```python
from build123d import *

# Parameters (mm, degrees)
BOSS_EXTRUDE1_DEPTH = 25.8


with BuildPart() as part:
    # Sketch1 → Boss-Extrude1 (new body)
    with BuildSketch(Plane.XZ.offset(25.8)):
        with BuildLine():
            Line((-0.494571956, -23.689779316), (-0.494571956, -23.589779316))
            Line((-0.494571956, -23.589779316), (-0.394571956, -23.589779316))
            Line((-0.394571956, -23.589779316), (33.993371563, -23.589779316))
            Line((33.993371563, -23.589779316), (38.063220374, -23.589779316))
            Line((38.063220374, -23.589779316), (37.29331502, -27.450677709))
            add(Edge.make_bspline(
                [(33.373472705, -47.107785962), (35.333393862, -37.279231836), (37.29331502, -27.450677709)],
                knots=[0, 0, 0, 1, 1, 1], degree=2))
            ThreePointArc((33.373472705, -47.107785962), (20.478962104, -86.002469597), (1.348099623, -122.238845235))
            Line((1.348099623, -122.238845235), (-0.494571956, -125.122735442))
            Line((-0.494571956, -125.122735442), (-0.494571956, -121.700417329))
            Line((-0.494571956, -121.700417329), (-0.494571956, -23.689779316))
        make_face()
        Polygon((1.636693568, -33.589779316), (31.180296724, -33.589779316), (28.552125449, -44.152877649), align=None, mode=Mode.SUBTRACT)
        with BuildLine():
            Line((1.8, -35.835600274), (27.903926427, -46.080219159))
            ThreePointArc((27.903926427, -46.080219159), (27.424243887, -48.283989571), (26.927669734, -50.484015362))
            Line((26.927669734, -50.484015362), (1.8, -38.383681926))
            Line((1.8, -38.383681926), (1.8, -35.835600274))
        make_face(mode=Mode.SUBTRACT)
        with BuildLine():
            Line((1.8, -40.603496686), (26.461878816, -52.479526576))
            ThreePointArc((26.461878816, -52.479526576), (25.912863392, -54.754715884), (25.345753049, -57.025462497))
            Line((25.345753049, -57.025462497), (1.8, -43.431924445))
            Line((1.8, -43.431924445), (1.8, -40.603496686))
        make_face(mode=Mode.SUBTRACT)
        with BuildLine():
            Line((1.8, -45.741299666), (24.827629624, -59.035712415))
            ThreePointArc((24.827629624, -59.035712415), (24.198120154, -61.402606851), (23.548915198, -63.764175052))
            Line((23.548915198, -63.764175052), (1.8, -48.936721812))
            Line((1.8, -48.936721812), (1.8, -45.741299666))
        make_face(mode=Mode.SUBTRACT)
        with BuildLine():
            Line((1.8, -51.35729301), (22.974243013, -65.792960045))
            ThreePointArc((22.974243013, -65.792960045), (22.250225593, -68.273323364), (21.504437212, -70.747227791))
            Line((21.504437212, -70.747227791), (1.8, -55.034267198))
            Line((1.8, -55.034267198), (1.8, -51.35729301))
        make_face(mode=Mode.SUBTRACT)
        with BuildLine():
            Line((1.8, -57.592312351), (20.868191148, -72.797909591))
            ThreePointArc((20.868191148, -72.797909591), (20.032066674, -75.415616602), (19.171511459, -78.02539415))
            Line((19.171511459, -78.02539415), (1.8, -61.907631839))
            Line((1.8, -61.907631839), (1.8, -57.592312351))
        make_face(mode=Mode.SUBTRACT)
        with BuildLine():
            Line((1.8, -63.544593475), (18.75085734, -79.272061417))
            ThreePointArc((18.75085734, -79.272061417), (17.733603559, -82.213523384), (16.685267787, -85.144051641))
            Line((16.685267787, -85.144051641), (1.8, -69.379364433))
            Line((1.8, -69.379364433), (1.8, -63.544593475))
        make_face(mode=Mode.SUBTRACT)
        with BuildLine():
            Line((1.8, -71.127270664), (16.223970717, -86.40340744))
            ThreePointArc((16.223970717, -86.40340744), (15.062552919, -89.498168213), (13.866413905, -92.579675475))
            Line((13.866413905, -92.579675475), (1.8, -77.977808183))
            Line((1.8, -77.977808183), (1.8, -71.127270664))
        make_face(mode=Mode.SUBTRACT)
        with BuildLine():
            Line((1.8, -79.861617911), (13.360943276, -93.851802636))
            ThreePointArc((13.360943276, -93.851802636), (12.031133738, -97.119012014), (10.66221999, -100.37003119))
            Line((10.66221999, -100.37003119), (1.8, -88.073893757))
            Line((1.8, -88.073893757), (1.8, -79.861617911))
        make_face(mode=Mode.SUBTRACT)
        with BuildLine():
            Line((1.8, -90.126243158), (10.108701369, -101.654385546))
            ThreePointArc((10.108701369, -101.654385546), (8.581699979, -105.113401186), (7.010340095, -108.552492716))
            Line((7.010340095, -108.552492716), (1.8, -100.212262217))
            Line((1.8, -100.212262217), (1.8, -90.126243158))
        make_face(mode=Mode.SUBTRACT)
        with BuildLine():
            Line((1.8, -102.47713769), (6.404592978, -109.847744231))
            ThreePointArc((6.404592978, -109.847744231), (4.143731804, -114.543136732), (1.8, -119.197717832))
            Line((1.8, -119.197717832), (1.8, -102.47713769))
        make_face(mode=Mode.SUBTRACT)
    extrude(amount=-BOSS_EXTRUDE1_DEPTH)


solid = part.part
```
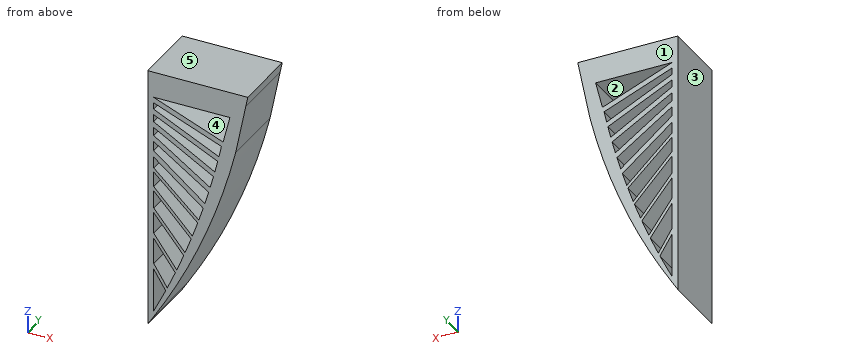
Geometry: final body of the model. Coordinates: model frame, mm. Face numbers are marked on the shaded views. A direction names the side the tool comes from. Round coordinates to 2 decimals unless told otherwise and drop trailing zeros. Order: outer loops, then holes, each group sorted by start corner. A loop starts at its lowest first (then second) coordinate and runs counter-clockwise, first axis right, second up. Notation, with made-up numbers: (70, 7.5) - (126, 7.5) arc R21 ccw to (126, 33.5) - close; hole circle Ø11 at (26.5, 89). An arc over 180 degrees is marked (long way). Use CSV: the item, a comma, the result in double quotes. Start each with the question number.
Q1. First-contact query: pin 1 (1.4 mm diameter, centred on y = -7.5, z = -42, fed in from +X); pin 2 (2 mm diameter, centred on y = -18.5, z = -37.5, fed in from +X); pin 3 (5.5 mm diameter, centred on y = -19.5, z = -76, fed in from +X); pin 4 (8 mm diameter, centred on x = 6, z = -50.5, fed in from +Y). Flat tips, straight axial feed; report the tip coordinate or a pass-through.
Q2. Section query A-A (x = 29.5). Return loops of the section in (y, z), and give its area (3 significant figures).
Q3. Mould query, pull axis X, two halves, no side actions, for the marked faces 3, 4 and 5. Classes: +X half, -X half, draft (parallel to the pull), parting line (faces both ways), or undercut.
Q4. Material intervals for line 1 along X through (y, z) = (-16.75, -97); line 2 along X through (y, z) = (-15.75, -66.5); line 3 along X through (y, z) = (-18, -94), sorted ascending. Write a range as from..to.
Q5. Section query B-B (z = -112.5). Return loops of the section in (x, y), and give its area (3 significant figures).
Q6. Section query D-D (y = -12.5). State how many separate pieces and enclosed holes the cut face has, and give its area (3 significant figures).
Q7. Section query C-C (z = -97.5). Return loops of the section in (x, y).
Q8. Access query for the marked faces 1 and 2. Directions: +Z, -Z, +X, -X, +Y, -Y. A direction counts if a zero-diameter tool reaches every point of the face in a straight line with its end or side. Return the directions, or none.
Result set:
1,pin 1,"stops at x = 34.53"
1,pin 2,"stops at x = 35.49"
1,pin 3,"stops at x = 25.5"
1,pin 4,"stops at y = 0"
2,outline,"(-25.8, -61.27) - (0, -61.27) - (0, -40.34) - (-25.8, -40.34) - close; (-25.8, -33.59) - (0, -33.59) - (0, -23.59) - (-25.8, -23.59) - close"
2,area,"798 mm2"
3,face 3,"-X half"
3,face 4,"undercut"
3,face 5,"draft"
4,line 1,"x = -0.49..1.8, 6.75..8.23, 12.08..15.47"
4,line 2,"x = -0.49..1.8, 4.99..6.75, 12.97..16.18, 22.77..27.84"
4,line 3,"x = -0.49..1.8, 4.59..6.07, 13.3..16.9"
5,outline,"(-0.49, -25.8) - (1.8, -25.8) - (1.8, 0) - (-0.49, 0) - close; (5.14, -25.8) - (7.26, -25.8) - (7.26, 0) - (5.14, 0) - close"
5,area,"114 mm2"
6,separate pieces,"1"
6,enclosed holes,"11"
6,area,"1,320 mm2"
7,outline,"(-0.49, -25.8) - (1.8, -25.8) - (1.8, 0) - (-0.49, 0) - close; (7.11, -25.8) - (8.59, -25.8) - (8.59, 0) - (7.11, 0) - close; (11.87, -25.8) - (15.23, -25.8) - (15.23, 0) - (11.87, 0) - close"
8,face 1,"+Z, -Z, +X, -X, +Y"
8,face 2,"+Y, -Y"
